Print and shaded views of the part. All mm, measured from the part's lowest x, y and z. A direction names the side the tool comes from. Coordinates: 2 decimals unless noted, no trailing zeros. Loops run counter-clockwise (first coordinate to the right, second up) from the corner with the lowest first, then second, coordinate; pieces in that order, holes last.
1) Pin check, flat tips, straight feed: pin 1 Ø2.5 at (x, y) = (10.5, 11.5) entering from +Z; pin 2 Ø4 at (x, z) = (2, 2) entering from +Y; pin 3 Ø8 at (y, z) = (4, 9.5) entering from +X. Stop position of each tip, or through.
2) Which spindle directions (+Z, -Z, +X, -X, +Y, -Y) get a long thin tool onto all of the face, cutting with end or side? Do the marked faces 1 and 2. Say none if no direction does.
3) Saw through at A-A, the plane y = 10. Write the cut outline in (x, z).
4) Two-plate mould, pull along Y, no slides. Class the marked faces 3, 4 and 5: +Y half, -Y half, draft (parallel to the pull), parting line (faces both ways), or undercut.
5) Saw through at C-C, the plane z = 12. Write the cut outline in (x, y), and give its area (3 significant figures).
6) Wall check: line 1 along Y through (x, z) = (10, 13.6); line 2 along Z through (x, y) = (9, 11.25); line 3 along X through (y, z) = (4.25, 1.5). Give the ranges that are in metal, low to high.
7) Saw through at D-D, the plane z = 2.25. Write the cut outline in (x, y), and give its area (3 significant figures).
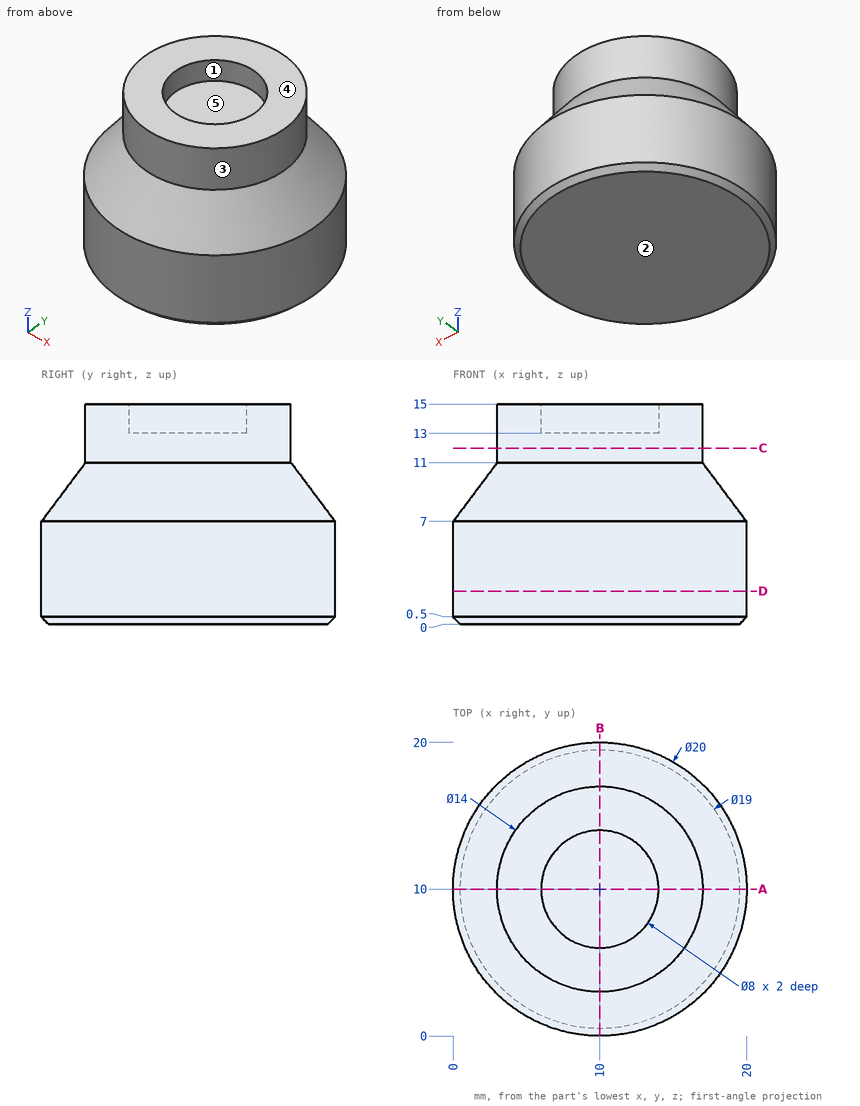
Data:
1. pin 1: stops at z = 13
1. pin 2: stops at y = 18
1. pin 3: stops at x = 19.58
2. face 1: +Z
2. face 2: -Z, +X, -X, +Y, -Y
3. outline: (0, 0.5) - (0.5, 0) - (19.5, 0) - (20, 0.5) - (20, 7) - (17, 11) - (17, 15) - (14, 15) - (14, 13) - (6, 13) - (6, 15) - (3, 15) - (3, 11) - (0, 7) - close
4. face 3: parting line
4. face 4: draft
4. face 5: undercut
5. outline: circle Ø14 at (10, 10)
5. area: 154 mm2
6. line 1: y = 3 to 6, 14 to 17
6. line 2: z = 0 to 13
6. line 3: x = 1.82 to 18.18
7. outline: circle Ø20 at (10, 10)
7. area: 314 mm2
